Here's how the part is built. I have some questions about the finished solid (model axes, mm). A direction names the side the tool comes from. Round coordinates to 2 decimals unless told otherwise and drop trailing zeros. Write each loop counter-clockwise with the first axis right and the second up, starting at its lowest first coordinate (ties: lowest second). Pieces come first, ordered by that corner, then holes. Notation, with made-up numbers: (8.5, -10) -> (57.5, -10) arc R23 ccw to (57.5, 11) -> close; hole circle Ø3 at (-39.75, -24). An arc over 180 degrees is marked (long way). Put each result on its own line as item: value. Start each with the question number.
1. For pin 1 (4 mm diameter, centred on x = 6.5, y = 27.5, fed in from +Z); pin 2 (6 mm diameter, centred on x = -15, z = 289.5, fed in from +Y); pin 3 (4 mm diameter, centred on x = -17.5, z = 16.5, fed in from -Y); pin 4 (10 mm diameter, centred on x = 15, z = 457, fed in from -Y), each with a flat end and sliding along its axis, tell me the tip position at first contact or that it passes through.
2. I need wall thicknesses on probe 1 along Z at (x, y) = (26, 31); probe 2 along Z at (x, y) = (-5, 13.5); probe 3 along Y at (x, z) = (18, 239.5). Which ranges of each line are inside material? Lowest first, please. Write a range as from..to.
3. Which directions (+Z, -Z, +X, -X, +Y, -Y) give clear straight access to the entire face, cutting with the end or side of a thin tool? Please do faces 4 (the face through (1, -32, 25.4)), 5 (the face through (-1, 25.4, 75)), 6 (the face through (-1, -38.1, 6)).
4. Suppose I cut it at D-D (x = 8.5). Please give me the cut outline in (y, z), then the cut area to 3 significant figures.
5. Suppose I cut it at A-A (x = -25). Please give me the cut outline in (y, z), then the cut area to 3 significant figures.
6. We'd pull the mould along Z, two halves only. Please class faces 1 (the face through (0.533, -28.044, 216.456)), 2 (the face through (1, -32, 12.7)), 3 (the face through (-1, 1, 0)): +Z half, -Z half, draft (parallel to the pull), parting line (faces both ways), or undercut.
7. Suppose I cut it at C-C (z = 176.5). Please give me the cut outline in (x, y).
8. Suppose I cut it at B-B (y = 7.5). Please give me the cut outline in (x, z), then the cut area to 3 significant figures.
```python
from build123d import *

# Parameters (mm, degrees)
F0_W      = 76.2
F0_H      = 76.2
F1_DEPTH  = 25.4
F2_W      = 76.2
F2_H      = 12.7
F3_DEPTH  = 101.6
F6_DEPTH  = 76.2
F7_W      = 12.7
F7_H      = 12.7
F8_DEPTH  = 76.201
F10_DEPTH = 59.1364003556
F12_DEPTH = 59.1364003556


with BuildPart() as f1:
    # F0 (on Top) → F1 (new body)
    with BuildSketch(Plane.XY):
        Rectangle(F0_W, F0_H)
    extrude(amount=F1_DEPTH)

    # F2 (on face) → F3 (join)
    with BuildSketch(Plane.XY.offset(25.4)):
        with Locations((0, 19.05)):
            Rectangle(F2_W, F2_H)
    extrude(amount=F3_DEPTH)

    # F5 (on face) → F6 (join, through all)
    with BuildSketch(Plane.YZ.offset(38.1)):
        Polygon((-38.1, 25.4), (12.7, 25.4), (12.7, 127), (-12.7, 508), align=None)
    extrude(amount=-F6_DEPTH)

    # F7 (on face) → F8 (cut, through all)
    with BuildSketch(Plane.YZ.offset(38.1)):
        with Locations((-31.75, 19.05)):
            Rectangle(F7_W, F7_H)
    extrude(amount=-F8_DEPTH, mode=Mode.SUBTRACT)

    # F9 (on face) → F10 (cut, through all)
    with BuildSketch(Plane(origin=(0, 21.0730088496, 1.4048672566), x_dir=(-1, 0, 0), z_dir=(0, 0.9977851579, 0.0665190105))):
        Polygon((-38.1, 125.8739236141), (0, 507.7196516248), (-38.1, 507.7196516248), align=None)
    extrude(amount=-F10_DEPTH, mode=Mode.SUBTRACT)

    # F11 (on face) → F12 (cut, through all)
    with BuildSketch(Plane(origin=(0, 21.0730088496, 1.4048672566), x_dir=(-1, 0, 0), z_dir=(0, 0.9977851579, 0.0665190105))):
        Polygon((38.1, 507.7196516248), (0, 507.7196516248), (38.1, 125.8739236141), align=None)
    extrude(amount=-F12_DEPTH, mode=Mode.SUBTRACT)


solid = f1.part
```
Verdict:
1. pin 1: stops at z = 25.4
1. pin 2: stops at y = 2.07
1. pin 3: stops at y = -25.4
1. pin 4: passes through
2. probe 1: z = 0..25.4
2. probe 2: z = 0..127
2. probe 3: y = -26.83..5.2
3. face 4: +X, -X, -Y
3. face 5: +Z, +X, -X, +Y
3. face 6: +Z, -Z, +X, -X, -Y
4. outline: (-38.1, 0) -> (38.1, 0) -> (38.1, 25.4) -> (25.4, 25.4) -> (25.4, 127) -> (12.7, 127) -> (-7.03, 423) -> (-17.21, 422.32) -> (-38.1, 25.4) -> (-25.4, 25.4) -> (-25.4, 12.7) -> (-38.1, 12.7) -> close
4. area: 16,200 mm^2
5. outline: (-38.1, 0) -> (38.1, 0) -> (38.1, 25.4) -> (25.4, 25.4) -> (25.4, 127) -> (12.7, 127) -> (3.97, 258) -> (-25.96, 256) -> (-38.1, 25.4) -> (-25.4, 25.4) -> (-25.4, 12.7) -> (-38.1, 12.7) -> close
5. area: 12,900 mm^2
6. face 1: +Z half
6. face 2: undercut
6. face 3: -Z half
7. outline: (-33.15, 9.4) -> (-32.89, -30.15) -> (32.89, -30.15) -> (33.15, 9.4) -> close
8. outline: (-38.1, 0) -> (38.1, 0) -> (38.1, 126.65) -> (30.3, 205) -> (-30.3, 205) -> (-38.1, 126.65) -> close
8. area: 15,000 mm^2
